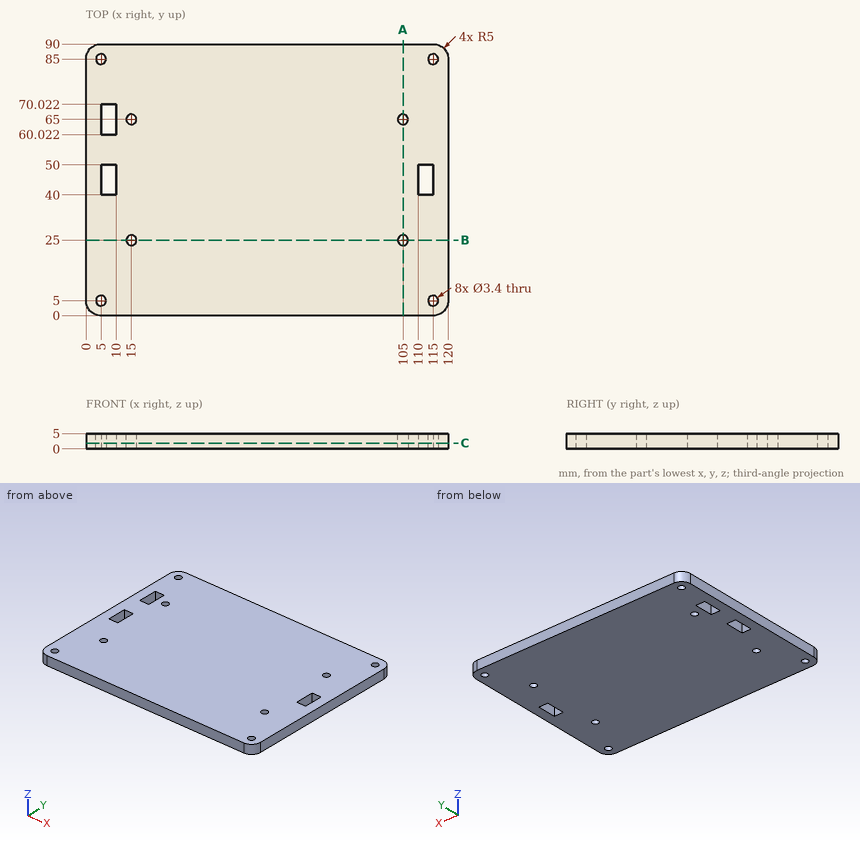
Geometry check sheet. Reference: drawing and pictorial views, mm from the part's lowest x, y, z. Round coordinates to 2 decimals unless told otherwise and drop trailing zeros. Order: outer loops, then holes, each group sorted by start corner. A loop starts at its lowest first (then second) coordinate and runs counter-clockwise, first axis right, second up. Notation, with made-up numbers: (74, 5.5) - (105, 5.5) arc R28 cw to (105, 23.5) - close; hole circle Ø7 at (-1, 45). An arc over 180 degrees is marked (long way). Use a Markdown table: item, result. Add a question column.
1) Section check A-A (x = 105). Record the cut outline in (y, z), then the cut area to 3 significant figures.
2) Thickness scan on line 1 along X through (y, z) = (41, 2.95); line 2 along X through (y, z) = (65, 2.65); line 3 along Y through (x, z) = (15, 3.65). Record the ranges inside material, lowest first.
3) Section check C-C (z = 1.9). Count the separate pieces of the cut face and the enclosed holes in it, then the cut area to 3 significant figures.
4) Section check B-B (y = 25). Record the cut outline in (x, z), then the cut area to 3 significant figures.
5) Gauge pin test, flat end, axial feed: P1, Ø2.5, axis at x = 115, y = 85, coming from the -Z side. Record the tip position at first contact, or that the pin passes through.
Established:
| question | item | result |
|---|---|---|
| 1 | outline | (0, 0) - (23.3, 0) - (23.3, 5) - (0, 5) - close; (26.7, 0) - (63.3, 0) - (63.3, 5) - (26.7, 5) - close; (66.7, 0) - (90, 0) - (90, 5) - (66.7, 5) - close |
| 1 | area | 416 mm2 |
| 2 | line 1 | 0 to 5, 10 to 110, 115 to 120 |
| 2 | line 2 | 0 to 5, 10 to 13.3, 16.7 to 103.3, 106.7 to 120 |
| 2 | line 3 | 0 to 23.3, 26.7 to 63.3, 66.7 to 90 |
| 3 | separate pieces | 1 |
| 3 | enclosed holes | 11 |
| 3 | area | 10,600 mm2 |
| 4 | outline | (0, 0) - (13.3, 0) - (13.3, 5) - (0, 5) - close; (16.7, 0) - (103.3, 0) - (103.3, 5) - (16.7, 5) - close; (106.7, 0) - (120, 0) - (120, 5) - (106.7, 5) - close |
| 4 | area | 566 mm2 |
| 5 | P1 | through |
